For this review, use the dimensioned drawing (mm, ordinates from the lowest corner) and the shaded views. Coordinates: 2 decimals unless noted, no trailing zeros. Order: outer loops, then holes, each group sorted by start corner. A loop starts at its lowest first (then second) coordinate and runs counter-clockwise, first axis right, second up. Notation, with made-up numbers: (83, 69.25) -> (141, 69.25) arc R10 ccw to (141, 78.25) -> close; hole circle Ø3 at (30.25, 36). An arc over 180 degrees is marked (long way). Use one line per item in the form item = value. Start each with the question number.
(1) Take a section at C-C (z = 30). State the section outline as (x, y) points.
(2) Mouldability with a two-part tool opening along X and no side actions: class the marked faces 1, 2 and 3 as +X half, -X half, draft (parallel to the pull), parting line (faces both ways), or undercut.
(3) Take a section at A-A (y = 3.5). State how many separate pieces and enclosed holes the cut face has, then the cut area to 3 significant figures.
(4) Take a section at B-B (x = 30). State the section outline as (y, z) points, then the cut area to 3 significant figures.
(5) Take a section at D-D (x = 9.7). State the section outline as (y, z) points, then the cut area to 3 significant figures.
(6) Wall thickness on line 1 along X through (y, z) = (7, 50.3); line 2 along X through (y, z) = (3.5, 30): over which ranges is each line inside the solid? List them lowest first.
(7) Insertion check: pin 1 Ø7 at (x, z) = (50.3, 9.7) entering from +Y. The pin has a flat end and moves straight along its axis. Give the tip position at first contact, or say it passes through.
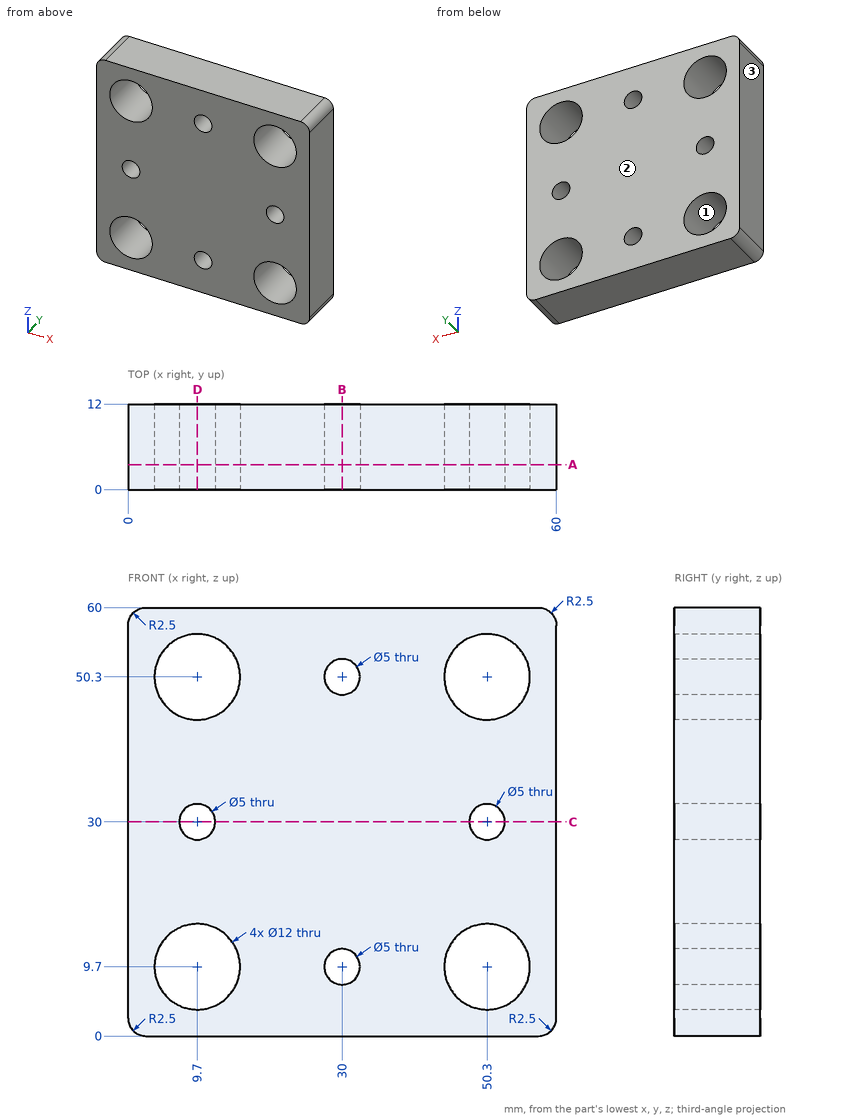
Findings:
q1.outline = (0, 0) -> (7.2, 0) -> (7.2, 12) -> (0, 12) -> close; (12.2, 0) -> (47.8, 0) -> (47.8, 12) -> (12.2, 12) -> close; (52.8, 0) -> (60, 0) -> (60, 12) -> (52.8, 12) -> close
q2.face_1 = undercut
q2.face_2 = draft
q2.face_3 = -X half
q3.separate_pieces = 1
q3.enclosed_holes = 8
q3.area = 3,060 mm²
q4.outline = (0, 0) -> (12, 0) -> (12, 7.2) -> (0, 7.2) -> close; (0, 12.2) -> (12, 12.2) -> (12, 47.8) -> (0, 47.8) -> close; (0, 52.8) -> (12, 52.8) -> (12, 60) -> (0, 60) -> close
q4.area = 600 mm²
q5.outline = (0, 0) -> (12, 0) -> (12, 3.7) -> (0, 3.7) -> close; (0, 15.7) -> (12, 15.7) -> (12, 27.5) -> (0, 27.5) -> close; (0, 32.5) -> (12, 32.5) -> (12, 44.3) -> (0, 44.3) -> close; (0, 56.3) -> (12, 56.3) -> (12, 60) -> (0, 60) -> close
q5.area = 372 mm²
q6.line_1 = 0 to 3.7, 15.7 to 27.5, 32.5 to 44.3, 56.3 to 60
q6.line_2 = 0 to 7.2, 12.2 to 47.8, 52.8 to 60
q7.pin_1 = through
